Input: dimensioned drawing with shaded views. Units: mm. Origin: part minimum x, y, z. Coordinates: 2 decimals unless noted, no trailing zeros. Order: outer loops, then holes, each group sorted by start corner. A loop starts at its lowest first (then second) coordinate and runs counter-clockwise, first axis right, second up. Notation, with made-up numbers: (86, 26) -> (132, 26) arc R11 cw to (132, 31) -> close; hole circle Ø10 at (71, 32). An arc over 180 degrees is marked (long way). Answer in a Markdown table with one row per item. Add a question column.
1) Section query A-A on y = 20. Return the cut outline in (x, z), then the cut area to 3 significant figures.
2) Ray query, line 1 (Z direction, x = 370, y = 21.5); line 2 (Y direction, x = 163, z = 25); line 3 (Z direction, x = 246.5, y = 25). Return the intervals inside material, ascending. Write a range as from..to.
3) Section query B-B on z = 281.5. Return the cut outline in (x, y), then the cut area to 3 significant figures.
4) Contact query for flat-ended pins moving along their axis: P1, Ø10, axis at y = 18.5, z = 81, coming from the +X side; P2, Ø3, axis at x = 334, z = 87, coming from the -Y side; P3, Ø1, axis at y = 34, z = 339, coming from the -X side. Output: stop coordinate, or through.
5) Section query C-C on x = 516. Return the cut outline in (y, z).
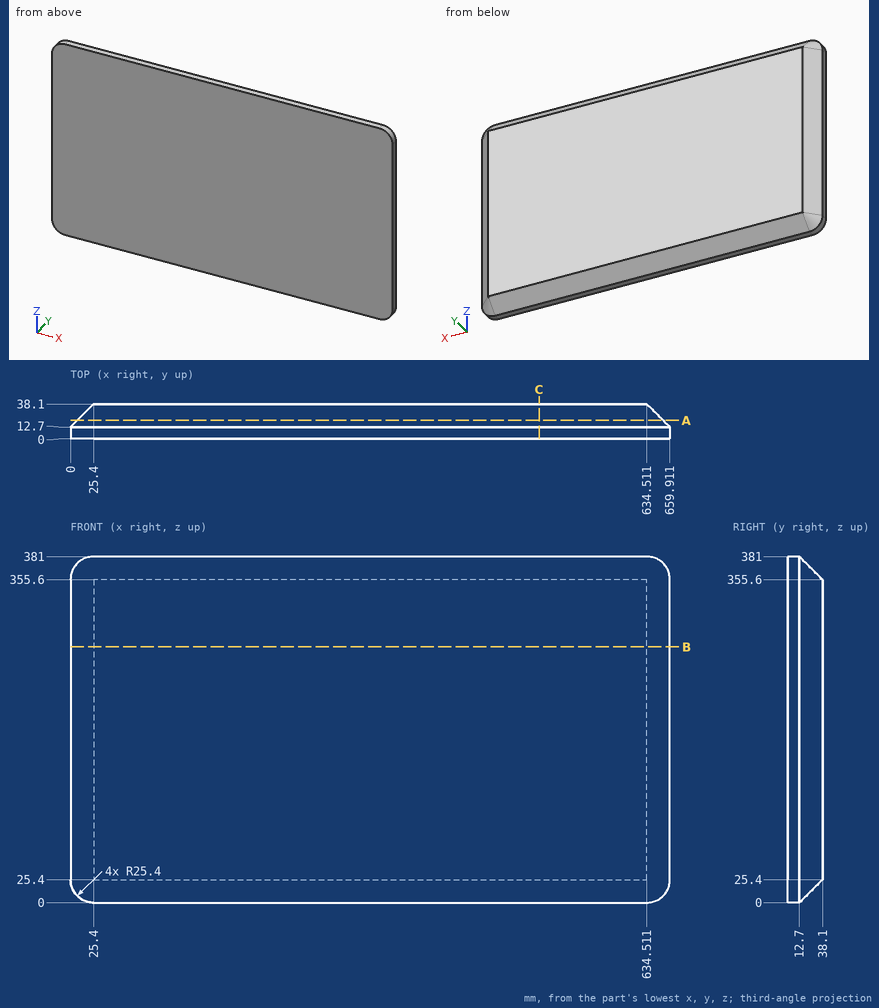
Result:
| question | item | result |
|---|---|---|
| 1 | outline | (7.3, 25.4) arc R18.1 ccw to (25.4, 7.3) -> (634.51, 7.3) arc R18.1 ccw to (652.61, 25.4) -> (652.61, 355.6) arc R18.1 ccw to (634.51, 373.7) -> (25.4, 373.7) arc R18.1 ccw to (7.3, 355.6) -> close |
| 1 | area | 236,000 mm2 |
| 2 | line 1 | 8.8..372.2 |
| 2 | line 2 | 0..37.7 |
| 2 | line 3 | 12.3..368.7 |
| 3 | outline | (0, 0) -> (659.91, 0) -> (659.91, 12.7) -> (634.51, 38.1) -> (25.4, 38.1) -> (0, 12.7) -> close |
| 3 | area | 24,500 mm2 |
| 4 | P1 | x = 659.11 |
| 4 | P2 | y = 0 |
| 4 | P3 | x = 20.8 |
| 5 | outline | (0, 0) -> (12.7, 0) -> (38.1, 25.4) -> (38.1, 355.6) -> (12.7, 381) -> (0, 381) -> close |
